Check sheet for the modelled part. Datum: model origin and axes. Units: mm. Coordinates: 2 decimals unless noted, no trailing zeros. Loops run counter-clockwise (first coordinate to the right, second up) from the corner with the lowest first, then second, coordinate; pieces in that order, holes last. Notation, with made-up numbers: (-14, 51) - (2, 51) arc R8 cw to (2, 56) - close; hole circle Ø9 at (-35, 31.25). An arc over 180 degrees is marked (long way). Use a Markdown table: item, result. Add a question column.
1) Thickness scan on line 1 (X direction, y = 0.75, z = -4.5); line 2 (X direction, y = 2.5, z = -1.25); line 3 (Z direction, x = 140.5, y = 1). Record the ranges inside material, lowest first.
2) Sectioned sample at B-B, the plane x = 294.5. Enter the section's corners in (y, z).
3) Sectioned sample at A-A, the plane z = 0. Enter the section's corners in (x, y) (1 decimal), then the cut area to 3 significant figures.
4) Go/stop test with flat-tipped pins: P1, Ø5, axis at x = 222, z = 2, coming from the +Y side; P2, Ø8, axis at y = 5, z = 1, coming from the +X side; P3, Ø5, axis at y = 7.5, z = 0.5, coming from the -X side. Record where each tip stops, or that it passes through.
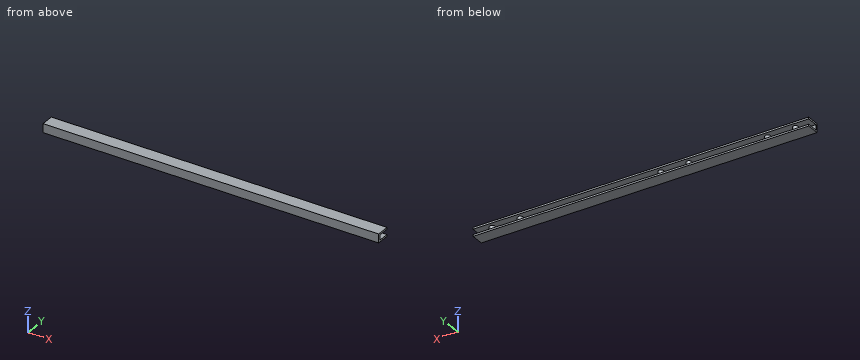
from build123d import *

# Parameters (mm, degrees)
BOSS_EXTRUDE1_DEPTH = 609.6
SKETCH2_R           = 4.7625
BOSS_EXTRUDE5_DEPTH = 9.525


with BuildPart() as part:
    # Sketch1 → Boss-Extrude1 (new body)
    with BuildSketch(Plane(origin=(0, 0, 0), x_dir=(0, 0, -1), z_dir=(1, 0, 0))):
        Polygon((-4.7625, 7.0485), (-4.7625, 11.7475), (-7.9375, 11.7475), (-7.9375, -11.7475), (7.9375, -11.7475), (7.9375, 11.7475), (4.7625, 11.7475), (4.7625, 8.5725), (4.7625, -8.5725), (-4.7625, -8.5725), align=None)
    extrude(amount=BOSS_EXTRUDE1_DEPTH)

    # Sketch2 → Boss-Extrude5 (add)
    with BuildSketch(Plane.XY.offset(4.7625)):
        with Locations((581.025, 1.5875)):
            Circle(SKETCH2_R)
        with Locations((530.225, 1.5875)):
            Circle(SKETCH2_R)
        with Locations((274.6375, 1.5875)):
            Circle(SKETCH2_R)
        with Locations((223.8375, 1.5875)):
            Circle(SKETCH2_R)
        with Locations((30.1625, 1.5875)):
            Circle(SKETCH2_R)
        with Locations((80.9625, 1.5875)):
            Circle(SKETCH2_R)
    extrude(amount=-BOSS_EXTRUDE5_DEPTH)


solid = part.part
Solved:
| question | item | result |
|---|---|---|
| 1 | line 1 | x = 25.47 to 34.85, 76.27 to 85.65, 219.15 to 228.53, 269.95 to 279.33, 525.54 to 534.91, 576.34 to 585.71 |
| 1 | line 2 | x = 25.49 to 34.84, 76.29 to 85.64, 219.16 to 228.51, 269.96 to 279.31, 525.55 to 534.9, 576.35 to 585.7 |
| 1 | line 3 | z = -7.94 to -4.76, 4.76 to 7.94 |
| 2 | outline | (-11.75, -7.94) - (11.75, -7.94) - (11.75, -4.76) - (-8.57, -4.76) - (-8.57, 4.76) - (11.75, 4.76) - (11.75, 7.94) - (-11.75, 7.94) - close |
| 3 | outline | (0, -11.7) - (609.6, -11.7) - (609.6, -8.6) - (0, -8.6) - close; circle Ø9.5 at (30.2, 1.6); circle Ø9.5 at (81, 1.6); circle Ø9.5 at (223.8, 1.6); circle Ø9.5 at (274.6, 1.6); circle Ø9.5 at (530.2, 1.6); circle Ø9.5 at (581, 1.6) |
| 3 | area | 2,360 mm2 |
| 4 | P1 | stops at y = 6.35 |
| 4 | P2 | stops at x = 609.6 |
| 4 | P3 | stops at x = 26.84 |
